from build123d import *

# Parameters (mm, degrees)
SKETCH1_W           = 28.15
SKETCH1_H           = 36.4
BOSS_EXTRUDE1_DEPTH = 10.26
SKETCH2_W           = 5.75
SKETCH2_H           = 22.86
SKETCH2_W_2         = 1.4
BOSS_EXTRUDE5_DEPTH = 7
BOSS_EXTRUDE6_DEPTH = 3
SKETCH5_R           = 1.5
SKETCH5_R_2         = 0.9
BOSS_EXTRUDE7_DEPTH = 12
BOSS_EXTRUDE8_DEPTH = 3
SKETCH8_R           = 1.5
SKETCH8_R_2         = 0.9
BOSS_EXTRUDE9_DEPTH = 12


with BuildPart() as part:
    # Sketch1 → Boss-Extrude1 (new body)
    with BuildSketch(Plane.XY):
        with Locations((-756.790122614, 155.279969002)):
            Rectangle(SKETCH1_W, SKETCH1_H)
    extrude(amount=BOSS_EXTRUDE1_DEPTH)

    # Sketch2 → Boss-Extrude5 (add)
    with BuildSketch(Plane.XY.offset(10.26)):
        with Locations((-759.219593617, 155.576927604)):
            Rectangle(SKETCH2_W, SKETCH2_H)
        with Locations((-753.644593617, 155.576927604)):
            Rectangle(SKETCH2_W_2, SKETCH2_H)
        with Locations((-749.580593617, 155.576927604)):
            Rectangle(SKETCH2_W_2, SKETCH2_H)
        with Locations((-747.548593617, 155.576927604)):
            Rectangle(SKETCH2_W_2, SKETCH2_H)
        with Locations((-751.612593617, 155.576927604)):
            Rectangle(SKETCH2_W_2, SKETCH2_H)
        with Locations((-764.936255693, 155.555778802)):
            Rectangle(SKETCH2_W_2, SKETCH2_H)
    extrude(amount=BOSS_EXTRUDE5_DEPTH)

    # Sketch4 → Boss-Extrude6 (add)
    with BuildSketch(Plane.XZ.offset(-144.146927604)):
        Polygon((-759.208791207, 11.000445338), (-756.524112455, 12.550445338), (-756.524112455, 15.650445338), (-759.208791207, 17.200445338), (-761.893469959, 15.650445338), (-761.893469959, 12.550445338), align=None)
    extrude(amount=BOSS_EXTRUDE6_DEPTH)

    # Sketch5 → Boss-Extrude7 (add)
    with BuildSketch(Plane.XZ.offset(-141.146927604)):
        with Locations(Location((-759.25539639, 14.147787096, 0), (0, 0, 270))):
            Circle(SKETCH5_R)
        with Locations(Location((-759.25539639, 14.147787096, 0), (0, 0, 270))):
            Circle(SKETCH5_R_2, mode=Mode.SUBTRACT)
    extrude(amount=BOSS_EXTRUDE7_DEPTH)

    # Sketch6 → Boss-Extrude8 (add)
    with BuildSketch(Plane(origin=(0, 167.006927604, 0), x_dir=(1, 0, 0), z_dir=(0, 1, 0))):
        Polygon((-759.16759572, -16.962225379), (-756.569519509, -15.462225379), (-756.569519509, -12.462225379), (-759.16759572, -10.962225379), (-761.765671931, -12.462225379), (-761.765671931, -15.462225379), align=None)
    extrude(amount=BOSS_EXTRUDE8_DEPTH)

    # Sketch8 → Boss-Extrude9 (add)
    with BuildSketch(Plane(origin=(0, 170.006927604, 0), x_dir=(1, 0, 0), z_dir=(0, 1, 0))):
        with Locations(Location((-759.042188193, -13.976282546, 0), (0, 0, 270))):
            Circle(SKETCH8_R)
        with Locations(Location((-759.042188193, -13.976282546, 0), (0, 0, 270))):
            Circle(SKETCH8_R_2, mode=Mode.SUBTRACT)
    extrude(amount=BOSS_EXTRUDE9_DEPTH)


solid = part.part
Verification items for the finished model (mm, model axes). A direction names the side the tool comes from. Coordinates: 2 decimals unless noted, no trailing zeros. Loops run counter-clockwise (first coordinate to the right, second up) from the corner with the lowest first, then second, coordinate; pieces in that order, holes last. Notation, with made-up numbers: M 85,-30.75 L 142,-30.75 A22 ccw 142,-17.75 Z; hole C 16.25,78.5 d11. An arc over 180 degrees is marked long. One line per item, written item: value.
1. Material ranges on line 1 along X through (y, z) = (150.5, 13.25); line 2 along Z through (x, y) = (-758.75, 173); line 3 along Y through (x, z) = (-758.5, 6.5), recorded low to high. Write a range as from..to.
Answers follow:
line 1: -765.64..-764.24, -762.09..-756.34, -754.34..-752.94, -752.31..-750.91, -750.28..-748.88, -748.25..-746.85
line 2: 0..10.26, 12.51..13.13, 14.83..15.45
line 3: 137.08..173.48
2. Section check A-A on z = 11.5. Give the number of separate pieces and of enclosed holes in the cut face, plus the area to 3 significant figures.
Answers follow:
separate pieces: 6
enclosed holes: 0
area: 302 mm^2
3. Set-up check for faces 1 (the flat face through (-752, 167.007, 14)), 2 (the cylindrical face through (-758.15, 175.92, 13.86)), 3 (the flat face through (-758, 141.147, 13)), 4 (the flat face through (-760.532, 142.668, 16.436)): record each of +Z, -Z, +X, -X, +Y, -Y from which the full face is reachable in a straight line by a thin tool's end or side.
Answers follow:
face 1: +Z, +X, +Y
face 2: +Y
face 3: -Y
face 4: +Z, -X, -Y
4. Section check C-C on y = 157.5. Record the cut outline in (x, z), plus the area to 3 significant figures.
Answers follow:
outline: M -770.87,0 L -742.72,0 L -742.72,10.26 L -746.85,10.26 L -746.85,17.26 L -748.25,17.26 L -748.25,10.26 L -748.88,10.26 L -748.88,17.26 L -750.28,17.26 L -750.28,10.26 L -750.91,10.26 L -750.91,17.26 L -752.31,17.26 L -752.31,10.26 L -752.94,10.26 L -752.94,17.26 L -754.34,17.26 L -754.34,10.26 L -756.34,10.26 L -756.34,17.26 L -762.09,17.26 L -762.09,10.26 L -764.24,10.26 L -764.24,17.26 L -765.64,17.26 L -765.64,10.26 L -770.87,10.26 Z
area: 378 mm^2
5. Section check D-D on x = -746. Record the cut outline in (y, z).
Answers follow:
outline: M 137.08,0 L 173.48,0 L 173.48,10.26 L 137.08,10.26 Z
6. Section check B-B on y = 140.5. Record the cut outline in (x, z), plus the area to 3 significant figures.
Answers follow:
outline: M -770.87,0 L -742.72,0 L -742.72,10.26 L -770.87,10.26 Z; C -759.26,14.15 d3; hole C -759.26,14.15 d1.8
area: 293 mm^2
7. Mould release check, pull along X, two halves, no side actions. Record for faces 5 (the flat face through (-748, 156, 17.26)), 6 (the flat face through (-750.913, 155, 14)), 7 (the flat face through (-770.865, 155, 5)): pulls with the +X half, pulls with the -X half, needs draft (parallel to the pull), parting line crosses it, or undercut.
Answers follow:
face 5: needs draft
face 6: undercut
face 7: pulls with the -X half
8. Gauge pin test, flat ends, axial feed: P1, Ø0.7, axis at x = -747, z = 12, coming from the +Y side; P2, Ø2, axis at x = -758, y = 140, coming from the +Z side; P3, Ø2, axis at y = 158.5, z = 15, coming from the -X side. Record the tip position at first contact, or that the pin passes through.
Answers follow:
P1: y = 167.01
P2: z = 15.63
P3: x = -765.64
